Could you check a few things on this model? Use its own coordinates, in mm. Give positions to 0.01 mm unless a question says otherwise; leave off trailing zeros. Order: outer loops, then holes, each group sorted by start corner. A loop starts at its lowest first (then second) coordinate and runs counter-clockwise, first axis right, second up. Notation, with made-up numbers: (-9.5, -22.5) -> (33.5, -22.5) arc R23 ccw to (33.5, 10.5) -> close; hole circle Ø8 at (36.5, -34). An arc over 180 degrees is marked (long way). Write each question's results on one line, items separated by ' | '.
```python
from build123d import *

# Parameters (mm, degrees)
F0_W      = 50
F0_H      = 40
F1_DEPTH  = 1.5
F2_W      = 50
F2_H      = 40
F3_DEPTH  = 10
F5_DEPTH  = 10
F7_DEPTH  = 10
F9_DEPTH  = 10
F11_DEPTH = 10
F14_W     = 1
F14_H     = 4.08333
F15_DEPTH = 6
F16_W     = 1
F16_H     = 0.2
F17_DEPTH = 2
F18_W     = 1
F18_H     = 3.60977
F19_DEPTH = 6
F20_W     = 1
F20_H     = 0.2
F21_DEPTH = 2
F22_W     = 1
F22_H     = 4.091013
F23_DEPTH = 6
F24_W     = 1
F24_H     = 0.2
F25_DEPTH = 2
F26_W     = 1
F26_H     = 3.330472
F27_DEPTH = 6
F28_W     = 1
F28_H     = 0.2
F29_DEPTH = 2
F30_W     = 1
F30_H     = 3.411457
F31_DEPTH = 6
F32_W     = 1
F32_H     = 0.2
F33_DEPTH = 2
F34_W     = 1
F34_H     = 3.646998
F35_DEPTH = 6
F36_W     = 1
F36_H     = 0.2
F37_DEPTH = 2


with BuildPart() as f1:
    # F0 (on Top) → F1 (new body)
    with BuildSketch(Plane.XY):
        with Locations((1.654343, -10.769538)):
            Rectangle(F0_W, F0_H)
    extrude(amount=F1_DEPTH)

    # F2 (on face) → F3 (join)
    with BuildSketch(Plane.XY.offset(1.5)):
        with Locations((1.654343, -10.769538)):
            Rectangle(F2_W, F2_H)
        Polygon((-21.845657, -29.269538), (-21.845657, 7.730462), (19.154343, 7.730462), (25.154343, 7.730462), (25.154343, 1.730462), (25.154343, -29.269538), align=None, mode=Mode.SUBTRACT)
    extrude(amount=F3_DEPTH)

    # F4 (on face) → F5 (join)
    with BuildSketch(Plane.XY.offset(1.5)):
        with BuildLine():
            Line((-20.083094, 5.967899), (-21.845657, 7.730462))
            Line((-21.845657, 7.730462), (-21.845657, 1.730462))
            Line((-21.845657, 1.730462), (-20.083094, 3.493025))
            ThreePointArc((-20.083094, 3.493025), (-20.595657, 4.730462), (-20.083094, 5.967899))
        make_face()
        with BuildLine():
            Line((-15.845657, 7.730462), (-21.845657, 7.730462))
            Line((-21.845657, 7.730462), (-20.083094, 5.967899))
            ThreePointArc((-20.083094, 5.967899), (-18.845657, 6.480462), (-17.60822, 5.967899))
            Line((-17.60822, 5.967899), (-15.845657, 7.730462))
        make_face()
        with BuildLine():
            Line((-15.845657, 1.730462), (-15.845657, 7.730462))
            Line((-15.845657, 7.730462), (-17.60822, 5.967899))
            ThreePointArc((-17.60822, 5.967899), (-17.228868, 5.400158), (-17.095657, 4.730462))
            ThreePointArc((-17.095657, 4.730462), (-17.228868, 4.060766), (-17.60822, 3.493025))
            Line((-17.60822, 3.493025), (-15.845657, 1.730462))
        make_face()
        with BuildLine():
            Line((-20.083094, 3.493025), (-21.845657, 1.730462))
            Line((-21.845657, 1.730462), (-15.845657, 1.730462))
            Line((-15.845657, 1.730462), (-17.60822, 3.493025))
            ThreePointArc((-17.60822, 3.493025), (-18.845657, 2.980462), (-20.083094, 3.493025))
        make_face()
    extrude(amount=F5_DEPTH)

    # F6 (on face) → F7 (join)
    with BuildSketch(Plane.XY.offset(1.5)):
        with BuildLine():
            Line((-20.083094, -27.506975), (-21.845657, -29.269538))
            Line((-21.845657, -29.269538), (-15.845657, -29.269538))
            Line((-15.845657, -29.269538), (-17.60822, -27.506975))
            ThreePointArc((-17.60822, -27.506975), (-18.845657, -28.019538), (-20.083094, -27.506975))
        make_face()
        with BuildLine():
            Line((-21.845657, -23.269538), (-21.845657, -29.269538))
            Line((-21.845657, -29.269538), (-20.083094, -27.506975))
            ThreePointArc((-20.083094, -27.506975), (-20.595657, -26.269538), (-20.083094, -25.032101))
            Line((-20.083094, -25.032101), (-21.845657, -23.269538))
        make_face()
        with BuildLine():
            Line((-17.60822, -27.506975), (-15.845657, -29.269538))
            Line((-15.845657, -29.269538), (-15.845657, -23.269538))
            Line((-15.845657, -23.269538), (-17.60822, -25.032101))
            ThreePointArc((-17.60822, -25.032101), (-17.228868, -25.599842), (-17.095657, -26.269538))
            ThreePointArc((-17.095657, -26.269538), (-17.228868, -26.939234), (-17.60822, -27.506975))
        make_face()
        with BuildLine():
            Line((-15.845657, -23.269538), (-21.845657, -23.269538))
            Line((-21.845657, -23.269538), (-20.083094, -25.032101))
            ThreePointArc((-20.083094, -25.032101), (-18.845657, -24.519538), (-17.60822, -25.032101))
            Line((-17.60822, -25.032101), (-15.845657, -23.269538))
        make_face()
    extrude(amount=F7_DEPTH)

    # F8 (on face) → F9 (join)
    with BuildSketch(Plane.XY.offset(1.5)):
        with BuildLine():
            Line((23.39178, 5.967899), (25.154343, 7.730462))
            Line((25.154343, 7.730462), (19.154343, 7.730462))
            Line((19.154343, 7.730462), (20.916906, 5.967899))
            ThreePointArc((20.916906, 5.967899), (22.154343, 6.480462), (23.39178, 5.967899))
        make_face()
        with BuildLine():
            Line((25.154343, 1.730462), (25.154343, 7.730462))
            Line((25.154343, 7.730462), (23.39178, 5.967899))
            ThreePointArc((23.39178, 5.967899), (23.771132, 5.400158), (23.904343, 4.730462))
            ThreePointArc((23.904343, 4.730462), (23.771132, 4.060766), (23.39178, 3.493025))
            Line((23.39178, 3.493025), (25.154343, 1.730462))
        make_face()
        with BuildLine():
            Line((20.916906, 5.967899), (19.154343, 7.730462))
            Line((19.154343, 7.730462), (19.154343, 1.730462))
            Line((19.154343, 1.730462), (20.916906, 3.493025))
            ThreePointArc((20.916906, 3.493025), (20.404343, 4.730462), (20.916906, 5.967899))
        make_face()
        with BuildLine():
            Line((19.154343, 1.730462), (25.154343, 1.730462))
            Line((25.154343, 1.730462), (23.39178, 3.493025))
            ThreePointArc((23.39178, 3.493025), (22.154343, 2.980462), (20.916906, 3.493025))
            Line((20.916906, 3.493025), (19.154343, 1.730462))
        make_face()
    extrude(amount=F9_DEPTH)

    # F10 (on face) → F11 (join)
    with BuildSketch(Plane.XY.offset(1.5)):
        with BuildLine():
            Line((23.39178, -27.506975), (25.154343, -29.269538))
            Line((25.154343, -29.269538), (25.154343, -23.269538))
            Line((25.154343, -23.269538), (23.39178, -25.032101))
            ThreePointArc((23.39178, -25.032101), (23.771132, -25.599842), (23.904343, -26.269538))
            ThreePointArc((23.904343, -26.269538), (23.771132, -26.939234), (23.39178, -27.506975))
        make_face()
        with BuildLine():
            Line((19.154343, -29.269538), (25.154343, -29.269538))
            Line((25.154343, -29.269538), (23.39178, -27.506975))
            ThreePointArc((23.39178, -27.506975), (22.154343, -28.019538), (20.916906, -27.506975))
            Line((20.916906, -27.506975), (19.154343, -29.269538))
        make_face()
        with BuildLine():
            Line((19.154343, -23.269538), (19.154343, -29.269538))
            Line((19.154343, -29.269538), (20.916906, -27.506975))
            ThreePointArc((20.916906, -27.506975), (20.404343, -26.269538), (20.916906, -25.032101))
            Line((20.916906, -25.032101), (19.154343, -23.269538))
        make_face()
        with BuildLine():
            Line((23.39178, -25.032101), (25.154343, -23.269538))
            Line((25.154343, -23.269538), (19.154343, -23.269538))
            Line((19.154343, -23.269538), (20.916906, -25.032101))
            ThreePointArc((20.916906, -25.032101), (22.154343, -24.519538), (23.39178, -25.032101))
        make_face()
    extrude(amount=F11_DEPTH)

    # F14 (on face) → F15 (join)
    with BuildSketch(Plane.XY.offset(1.5)):
        with Locations((15.880012, -2.9618)):
            Rectangle(F14_W, F14_H)
    extrude(amount=F15_DEPTH)

    # F16 (on face) → F17 (cut)
    with BuildSketch(Plane.XY.offset(7.5)):
        with Locations((15.880012, -2.8618)):
            Rectangle(F16_W, F16_H)
    extrude(amount=-F17_DEPTH, mode=Mode.SUBTRACT)

    # F18 (on face) → F19 (join)
    with BuildSketch(Plane.XY.offset(1.5)):
        with Locations((15.880012, -16.79546)):
            Rectangle(F18_W, F18_H)
    extrude(amount=F19_DEPTH)

    # F20 (on face) → F21 (cut)
    with BuildSketch(Plane.XY.offset(7.5)):
        with Locations((15.880012, -16.945772)):
            Rectangle(F20_W, F20_H)
    extrude(amount=-F21_DEPTH, mode=Mode.SUBTRACT)

    # F22 (on face) → F23 (join)
    with BuildSketch(Plane.XY.offset(1.5)):
        with Locations((7.957027, -2.965641)):
            Rectangle(F22_W, F22_H)
    extrude(amount=F23_DEPTH)

    # F24 (on face) → F25 (cut)
    with BuildSketch(Plane.XY.offset(7.5)):
        with Locations((7.957027, -2.865641)):
            Rectangle(F24_W, F24_H)
    extrude(amount=-F25_DEPTH, mode=Mode.SUBTRACT)

    # F26 (on face) → F27 (join)
    with BuildSketch(Plane.XY.offset(1.5)):
        with Locations((8.577565, -16.655811)):
            Rectangle(F26_W, F26_H)
    extrude(amount=F27_DEPTH)

    # F28 (on face) → F29 (cut)
    with BuildSketch(Plane.XY.offset(7.5)):
        with Locations((8.577565, -16.555811)):
            Rectangle(F28_W, F28_H)
    extrude(amount=-F29_DEPTH, mode=Mode.SUBTRACT)

    # F30 (on face) → F31 (join)
    with BuildSketch(Plane.XY.offset(1.5)):
        with Locations((-2.510325, -10.103692)):
            Rectangle(F30_W, F30_H)
    extrude(amount=F31_DEPTH)

    # F32 (on face) → F33 (cut)
    with BuildSketch(Plane.XY.offset(7.5)):
        with Locations((-2.510325, -10.003692)):
            Rectangle(F32_W, F32_H)
    extrude(amount=-F33_DEPTH, mode=Mode.SUBTRACT)

    # F34 (on face) → F35 (join)
    with BuildSketch(Plane.XY.offset(1.5)):
        with Locations((-8.459517, -10.221463)):
            Rectangle(F34_W, F34_H)
    extrude(amount=F35_DEPTH)

    # F36 (on face) → F37 (cut)
    with BuildSketch(Plane.XY.offset(7.5)):
        with Locations((-8.459517, -10.121463)):
            Rectangle(F36_W, F36_H)
    extrude(amount=-F37_DEPTH, mode=Mode.SUBTRACT)


with BuildPart() as f12_1:
    # F12: copy of F1
    add(f1.part)


solid = f1.part
```
Q1. Suppose I cut it at B-B on z = 2.5. State how many separate pieces and enclosed holes the cut face has, and give its area (3 significant figures).
Here are the results:
separate pieces: 7 | enclosed holes: 5 | area: 389 mm²
Q2. Suppose I cut it at A-A on x = -14. Please give me the cut outline in (y, z), and give its area (3 significant figures).
Here are the results:
outline: (-30.77, 0) -> (9.23, 0) -> (9.23, 11.5) -> (7.73, 11.5) -> (7.73, 1.5) -> (-29.27, 1.5) -> (-29.27, 11.5) -> (-30.77, 11.5) -> close | area: 90.0 mm²
Q3. I'm going to push flat-ended pins straight in: pin 1 Ø1.8 at (x, y) = (21.5, 4.5) entering from +Z; pin 2 Ø0.5 at (x, y) = (-2.5, -9) entering from +Z. Where does each tip first touch, or does it pass through?
Here are the results:
pin 1: stops at z = 1.5 | pin 2: stops at z = 7.5
Q4. Suppose I cut it at C-C on y = -14. Please give me the cut outline in (x, z), and give its area (3 significant figures).
Here are the results:
outline: (-23.35, 0) -> (26.65, 0) -> (26.65, 11.5) -> (25.15, 11.5) -> (25.15, 1.5) -> (-21.85, 1.5) -> (-21.85, 11.5) -> (-23.35, 11.5) -> close | area: 105 mm²
Q5. I need wall thicknesses on line 1 along X through (y, z) = (-10.5, 5.75); line 2 along X through (y, z) = (-2, 6); line 3 along Y through (x, z) = (9, 4.75). Which ranges of each line are inside material? Lowest first, please.
Here are the results:
line 1: x = -23.35 to -21.85, -8.96 to -7.96, -3.01 to -2.01, 25.15 to 26.65 | line 2: x = -23.35 to -21.85, 7.46 to 8.46, 15.38 to 16.38, 25.15 to 26.65 | line 3: y = -30.77 to -29.27, -18.32 to -14.99, 7.73 to 9.23
